Source: CAD feature listing. Evaluate the final solid. Frame: model axes, mm. A direction names the side the tool comes from. Give positions to 0.01 mm unless a question says otherwise; leave off trailing zeros. Loops run counter-clockwise (first coordinate to the right, second up) from the corner with the lowest first, then second, coordinate; pieces in that order, holes last.
from build123d import *

# Parameters (mm, degrees)
SCHNITT_LINEAR_AUSTRAGEN1_DEPTH = 1.8
FASE1_SIZE                      = 0.2
VERRUNDUNG1_R                   = 0.2
VERRUNDUNG2_R                   = 0.1


with BuildPart() as part:
    # Skizze1 → Rotation1 (revolve)
    with BuildSketch(Plane(origin=(0, 0, 0), x_dir=(0, 0, -1), z_dir=(1, 0, 0))):
        Polygon((-3, 0), (-3, 2.75), (0, 2.75), (0, 1.465), (8, 1.465), (8, 0), align=None)
    revolve(axis=Axis((0, 0, 21.919879518), (0, 0, -1)))

    # Skizze2 → Schnitt-Linear austragen1 (cut)
    with BuildSketch(Plane.XY.offset(3)):
        Polygon((1.25, -0.721687836), (1.25, 0.721687836), (0, 1.443375673), (-1.25, 0.721687836), (-1.25, -0.721687836), (0, -1.443375673), align=None)
    extrude(amount=-SCHNITT_LINEAR_AUSTRAGEN1_DEPTH, mode=Mode.SUBTRACT)

    # Fase1
    fase1_edges = [part.edges().sort_by_distance(p)[0] for p in [
        (0, -1.465, -8),
        (0, -2.75, 0),
        (0, -2.75, 3),
    ]]
    chamfer(fase1_edges, length=FASE1_SIZE)

    # Verrundung1
    verrundung1_edges = [part.edges().sort_by_distance(p)[0] for p in [
        (0.625, -1.082531755, 1.2),
        (1.25, -0.721687836, 2.1),
        (-0.625, -1.082531755, 1.2),
        (0, -1.443375673, 2.1),
        (-1.25, 0, 1.2),
        (-1.25, -0.721687836, 2.1),
        (-0.625, 1.082531755, 1.2),
        (-1.25, 0.721687836, 2.1),
        (0.625, 1.082531755, 1.2),
        (0, 1.443375673, 2.1),
        (1.25, 0, 1.2),
        (1.25, 0.721687836, 2.1),
        (0, -1.465, 0),
    ]]
    fillet(verrundung1_edges, radius=VERRUNDUNG1_R)

    # Verrundung2
    verrundung2_edges = [part.edges().sort_by_distance(p)[0] for p in [
        (-0.625, -1.082531755, 3),
        (-1.25, 0, 3),
        (-0.625, 1.082531755, 3),
        (0.625, 1.082531755, 3),
        (1.25, 0, 3),
        (0.625, -1.082531755, 3),
        (-1.223205081, -0.706217783, 3),
        (0, -1.412435565, 3),
        (1.223205081, -0.706217783, 3),
        (1.223205081, 0.706217783, 3),
        (0, 1.412435565, 3),
        (-1.223205081, 0.706217783, 3),
    ]]
    fillet(verrundung2_edges, radius=VERRUNDUNG2_R)


solid = part.part
1) Cut plane A-A (y = 0). Return loops of the section in (x, z) (3 decimals).
Checks:
outline: (-2.75, 0.2) - (-2.55, 0) - (-1.665, 0) arc R0.2 cw to (-1.465, -0.2) - (-1.465, -7.8) - (-1.265, -8) - (1.265, -8) - (1.465, -7.8) - (1.465, -0.2) arc R0.2 cw to (1.665, 0) - (2.55, 0) - (2.75, 0.2) - (2.75, 2.8) - (2.55, 3) - (1.35, 3) arc R0.1 ccw to (1.25, 2.9) - (1.25, 1.4) arc R0.2 cw to (1.05, 1.2) - (-1.05, 1.2) arc R0.2 cw to (-1.25, 1.4) - (-1.25, 2.9) arc R0.1 ccw to (-1.35, 3) - (-2.55, 3) - (-2.75, 2.8) - close
2) Reachability of faces 1 (the flat face through (0, 0, 1.2)), 2 (the cylindrical face through (-1.43, -0.32, -4.05)), 3 (the flat face through (-1.1, -1.1, 3)) from +Z, -Z, +X, -X, +Y, -Y: full face, straight path, thin tool, end or side. Return the list, or none.
Checks:
face 1: +Z
face 2: -Z
face 3: +Z, +X, -X, +Y, -Y
3) Ray query, probe 1 along Z at (x, y) = (1.7, 1.6); probe 2 along X at (y, z) = (1.1, 1.5); probe 3 along Z at (x, y) = (-0.5, 0.65). Return the intervals inside material, ascending.
Checks:
probe 1: z = 0 to 3
probe 2: x = -2.52 to -0.59, 0.59 to 2.52
probe 3: z = -8 to 1.2
4) Cut plane B-B (z = -4.5). Return loops of the section in (x, y) (3 decimals).
Checks:
outline: circle Ø2.93 at (0, 0)
5) Contact query for flat-ended pins moving along their axis: P1, Ø2, axis at x = 1, z = -3, coming from the +Y side (3 decimals); P2, Ø2, axis at y = 0.5, z = -4.5, coming from the -X side (3 decimals); P3, Ø1.5, axis at x = 0.5, z = -3, coming from the -Y side (3 decimals). Output: stop coordinate, or through.
Checks:
P1: stops at y = 1.465
P2: stops at x = -1.465
P3: stops at y = -1.465
6) Pull-direction query (X, two-part tool) for faces 4 (the flat face through (-1, 2, 0)), 5 (the flat face through (1.25, 0, 2)), 6 (the cylindrical face through (-2.685, -0.596, 1.482)); classes: released by +X, released by -X, zero draft, split by the parting line, or undercut.
Checks:
face 4: zero draft
face 5: undercut
face 6: split by the parting line
